Input: dimensioned drawing with shaded views. Units: mm. Origin: part minimum x, y, z. A direction names the side the tool comes from. Coordinates: 2 decimals unless noted, no trailing zeros. Order: outer loops, then holes, each group sorted by start corner. A loop starts at its lowest first (then second) coordinate and runs counter-clockwise, first axis right, second up. Notation, with made-up numbers: (28.25, -24) - (46.25, -24) arc R14 cw to (46.25, -18) - close; hole circle Ø2 at (32.5, -6.5). An arc over 180 degrees is marked (long way). One line per question, with ' | ' between items. Start each with the question number.
(1) Draft query along X for the marked faces 1, 2, 3 and 4. Return one class per face: +X half, -X half, draft (parallel to the pull), parting line (faces both ways), or undercut.
(2) Section B-B (y = 57.5). Return the cut outline in (x, z), then the cut area to 3 significant figures.
(3) Contact query for flat-ended pins moving along their axis: P1, Ø5, axis at x = 22.5, z = 27.5, coming from the +Y side; P2, Ø5, axis at x = 15, y = 25.5, coming from the -Z side; P3, Ø12.5, axis at x = 26, y = 49, coming from the +Z side. Output: stop coordinate, or through.
(4) Section C-C (z = 92). Return the cut outline in (x, y), then the cut area to 3 significant figures.
(5) Line query: line 1 along Y through (x, z) = (16, 144); line 2 along X through (y, z) = (73, 19); line 3 along Z through (x, y) = (10, 18). Output: solid intervals per line, ascending.
(6) Section D-D (y = 31.5). Return the cut outline in (x, z).
(7) Access query for the marked faces 5, 6, 7 and 8. Directions: +Z, -Z, +X, -X, +Y, -Y. A direction counts if a zero-diameter tool reaches every point of the face in a straight line with its end or side. Return the directions, or none.
(8) Section A-A (x = 27.5). Return the cut outline in (y, z).
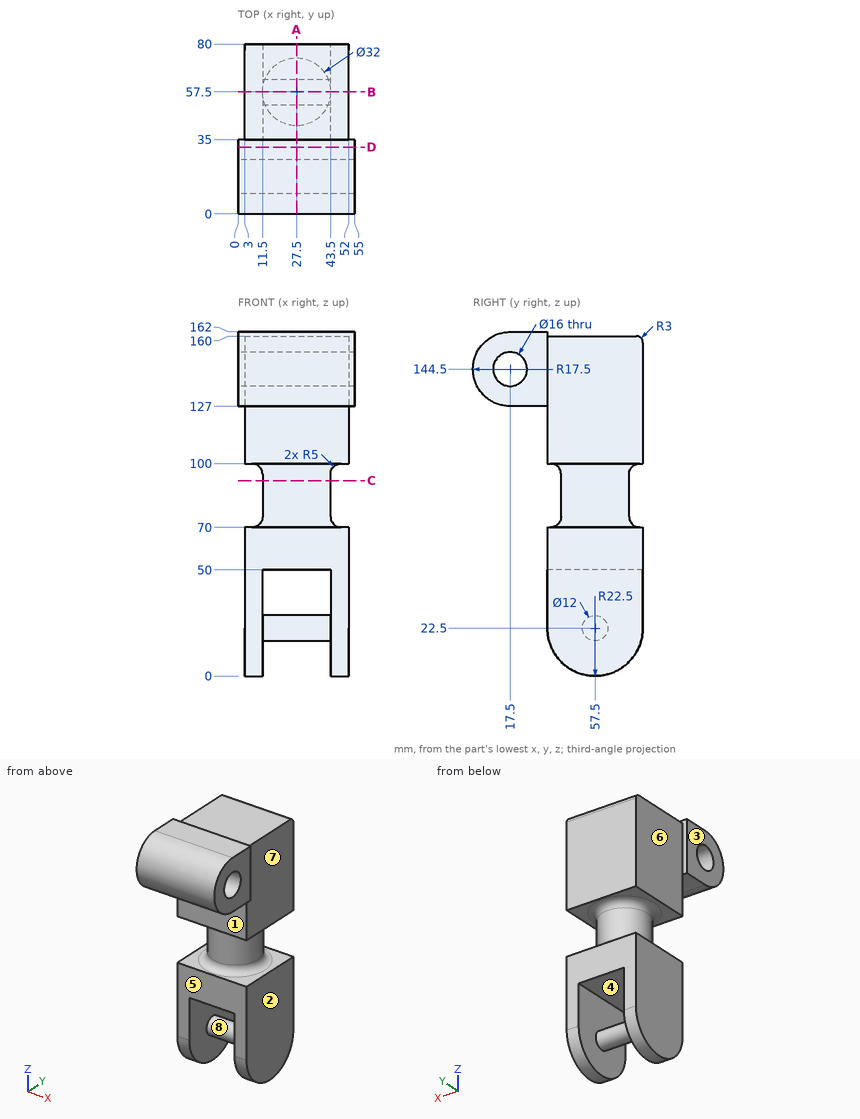
Response values:
1) face 1: draft | face 2: +X half | face 3: -X half | face 4: undercut
2) outline: (3, 0) - (11.5, 0) - (11.5, 16.5) - (43.5, 16.5) - (43.5, 0) - (52, 0) - (52, 70) - (48.5, 70) arc R5 cw to (43.5, 75) - (43.5, 95) arc R5 cw to (48.5, 100) - (52, 100) - (52, 160) - (3, 160) - (3, 100) - (6.5, 100) arc R5 cw to (11.5, 95) - (11.5, 75) arc R5 cw to (6.5, 70) - (3, 70) - close; hole (11.5, 28.5) - (43.5, 28.5) - (43.5, 50) - (11.5, 50) - close | area: 6,140 mm²
3) P1: stops at y = 62.95 | P2: stops at z = 127 | P3: stops at z = 160
4) outline: circle Ø32 at (27.5, 57.5) | area: 804 mm²
5) line 1: y = 0.01 to 9.52, 25.48 to 80 | line 2: x = 3 to 11.5, 43.5 to 52 | line 3: z = 127 to 136.52, 152.48 to 162
6) outline: (0, 127) - (55, 127) - (55, 162) - (0, 162) - close
7) face 5: -Z, +X, -X, -Y | face 6: +Z, -Z, -X, +Y | face 7: +Z, -Z, +X, +Y | face 8: none
8) outline: (17.5, 127) - (35, 127) - (35, 100) - (36.5, 100) arc R5 cw to (41.5, 95) - (41.5, 75) arc R5 cw to (36.5, 70) - (35, 70) - (35, 50) - (80, 50) - (80, 70) - (78.5, 70) arc R5 cw to (73.5, 75) - (73.5, 95) arc R5 cw to (78.5, 100) - (80, 100) - (80, 157) arc R3 ccw to (77, 160) - (35, 160) - (35, 162) - (17.5, 162) arc R17.5 ccw to start; circle Ø12 at (57.5, 22.5); hole circle Ø16 at (17.5, 144.5)
